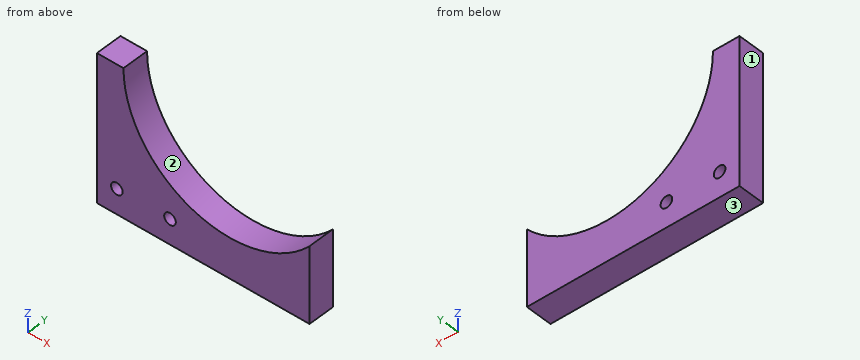
```python
from build123d import *

# Parameters (mm, degrees)
SKETCH1_W           = 304.8
SKETCH1_H           = 304.8
BOSS_EXTRUDE1_DEPTH = 6.35
CUT_EXTRUDE1_DEPTH  = 432.099063441
SKETCH3_R           = 25.4
CUT_EXTRUDE2_DEPTH  = 310.0695755
SKETCH4_R           = 1.3890625
CUT_EXTRUDE3_DEPTH  = 310.0695755


with BuildPart() as part:
    # Sketch1 → Boss-Extrude1 (new body)
    with BuildSketch(Plane(origin=(0, 0, 0), x_dir=(1, 0, 0), z_dir=(0, 1, 0))):
        with Locations((152.4, 152.4)):
            Rectangle(SKETCH1_W, SKETCH1_H)
    extrude(amount=BOSS_EXTRUDE1_DEPTH)

    # Sketch2 → Cut-Extrude1 (cut, through all)
    with BuildSketch(Plane(origin=(0, 6.35, 0), x_dir=(1, 0, 0), z_dir=(0, 1, 0))):
        Polygon((50.8, 304.8), (50.8, 269.875), (0, 269.875), (0, 0), (304.8, 0), (304.8, 304.8), align=None)
    extrude(amount=-CUT_EXTRUDE1_DEPTH, mode=Mode.SUBTRACT)

    # Sketch3 → Cut-Extrude2 (cut, through all)
    with BuildSketch(Plane(origin=(0, 6.35, 0), x_dir=(1, 0, 0), z_dir=(0, 1, 0))):
        with Locations((31.75, 269.875)):
            Circle(SKETCH3_R)
    extrude(amount=-CUT_EXTRUDE2_DEPTH, mode=Mode.SUBTRACT)

    # Sketch4 → Cut-Extrude3 (cut, through all)
    with BuildSketch(Plane(origin=(0, 6.35, 0), x_dir=(1, 0, 0), z_dir=(0, 1, 0))):
        with Locations(Location((4.7625, 298.833465882, 0), (0, 0, 270))):
            Circle(SKETCH4_R)
        with Locations(Location((17.4625, 298.833465882, 0), (0, 0, 270))):
            Circle(SKETCH4_R)
    extrude(amount=-CUT_EXTRUDE3_DEPTH, mode=Mode.SUBTRACT)


solid = part.part
```
For this review, take the finished solid that the model builds, in its own axes (mm). Face numbers are marked on the shaded views. Round coordinates to 2 decimals unless told otherwise and drop trailing zeros. Write each loop counter-clockwise with the first axis right and the second up, starting at its lowest first coordinate (ties: lowest second). Pieces come first, ordered by that corner, then holes. Notation, with made-up numbers: (-4.5, 52) - (26.5, 52) arc R7 cw to (26.5, 63) - close; hole circle Ø6 at (56, 89). An arc over 180 degrees is marked (long way). Answer as a JSON object with one key per item and string values.
1. We need section C-C on x = 18. Give the boundary of the cut face in (y, z), then the cut area to 3 significant figures.
Response values:
{"outline": "(0, -304.8) - (6.35, -304.8) - (6.35, -300.11) - (0, -300.11) - close; (0, -297.55) - (6.35, -297.55) - (6.35, -291.23) - (0, -291.23) - close", "area": "69.9 mm2"}
2. For pin 1 Ø3 at (x, y) = (42.5, 0.5) entering from +Z, flat-tipped, find the tip position at first contact; note if it passes through.
Response values:
{"pin 1": "stops at z = -292.13"}
3. We need section D-D on z = -299.5. Give the boundary of the cut face in (x, y).
Response values:
{"outline": "(0, 0) - (3.54, 0) - (3.54, 6.35) - (0, 6.35) - close; (5.98, 0) - (16.24, 0) - (16.24, 6.35) - (5.98, 6.35) - close; (18.68, 0) - (50.8, 0) - (50.8, 6.35) - (18.68, 6.35) - close"}
4. Draft analysis for pull direction X (two halves, no side actions). For the marked faces 1, 2 and 3, state which applies: +X half, -X half, draft (parallel to the pull), parting line (faces both ways), or undercut.
Response values:
{"face 1": "-X half", "face 2": "undercut", "face 3": "draft"}
5. To check wall thickness, follow line 1 along X through (y, z) = (0.75, -299.5); line 2 along Z through (x, y) = (32, 6.25); line 3 along Z through (x, y) = (17.5, 0.75). State the ranges of each line that lie inside material, in increasing order.
Response values:
{"line 1": "x = 0 to 3.54, 5.98 to 16.24, 18.68 to 50.8", "line 2": "z = -304.8 to -295.27", "line 3": "z = -304.8 to -300.22, -297.44 to -290.9"}
6. We need section B-B on y = 4.25. Count the separate pieces of the cut face and the enclosed holes in it, then the cut area to 3 significant figures.
Response values:
{"separate pieces": "1", "enclosed holes": "2", "area": "822 mm2"}
7. We need section A-A on z = -289.5. Give the boundary of the cut face in (x, y), then the cut area to 3 significant figures.
Response values:
{"outline": "(0, 0) - (15.62, 0) - (15.62, 6.35) - (0, 6.35) - close; (47.88, 0) - (50.8, 0) - (50.8, 6.35) - (47.88, 6.35) - close", "area": "118 mm2"}
